Part model, mm, in its own coordinate system. Give positions to 0.01 mm unless a question says otherwise; leave off trailing zeros. Order: outer loops, then holes, each group sorted by start corner. A loop starts at its lowest first (then second) coordinate and runs counter-clockwise, first axis right, second up.
1. Slice it at C-C on y = 235.3. List the corners of the cut face in (x, z), and give its area (3 significant figures).
2. Slice it at B-B on x = -9.25. List the corners of the cut face in (y, z) (3 decimals).
3. Slice it at D-D on x = 18.5. List the corners of the cut face in (y, z) (3 decimals).
4. Drop flat-ended pins along their axis: pin 1 Ø1 at (x, y) = (-17, 235) entering from -Z; pin 2 Ø12 at (x, z) = (-7.5, 15.5) entering from +Y; pin 3 Ø1 at (x, y) = (-5.5, 234.5) entering from +Z. Give the stop position or say it passes through.
5. Slice it at A-A on z = 0. List the corners of the cut face in (x, y) (3 decimals).
6. Probe line 1 (X direction, y = 233.7, z = -1.5); line 2 (X direction, y = 235.85, z = -18); line 3 (Z direction, x = 11, y = 235.1). List the from-to ranges inside material, lowest first.
from build123d import *

# Parameters (mm, degrees)
SKETCH2_R           = 22.5
SKETCH2_R_2         = 2.25
BOSS_EXTRUDE1_DEPTH = 3.175


with BuildPart() as part:
    # Sketch2 → Boss-Extrude1 (new body)
    with BuildSketch(Plane(origin=(0, 236.49, 0), x_dir=(1, 0, 0), z_dir=(0, 1, 0))):
        with Locations(Location((0, 0, 0), (0, 0, 270))):
            Circle(SKETCH2_R)
        with Locations(Location((9.25, 16.02146997, 0), (0, 0, 270))):
            Circle(SKETCH2_R_2, mode=Mode.SUBTRACT)
        with Locations(Location((18.5, 0, 0), (0, 0, 270))):
            Circle(SKETCH2_R_2, mode=Mode.SUBTRACT)
        with Locations(Location((9.25, -16.02146997, 0), (0, 0, 270))):
            Circle(SKETCH2_R_2, mode=Mode.SUBTRACT)
        with Locations(Location((-9.25, -16.02146997, 0), (0, 0, 270))):
            Circle(SKETCH2_R_2, mode=Mode.SUBTRACT)
        with Locations(Location((-18.5, 0, 0), (0, 0, 270))):
            Circle(SKETCH2_R_2, mode=Mode.SUBTRACT)
        with Locations(Location((-9.25, 16.02146997, 0), (0, 0, 270))):
            Circle(SKETCH2_R_2, mode=Mode.SUBTRACT)
    extrude(amount=-BOSS_EXTRUDE1_DEPTH)


solid = part.part
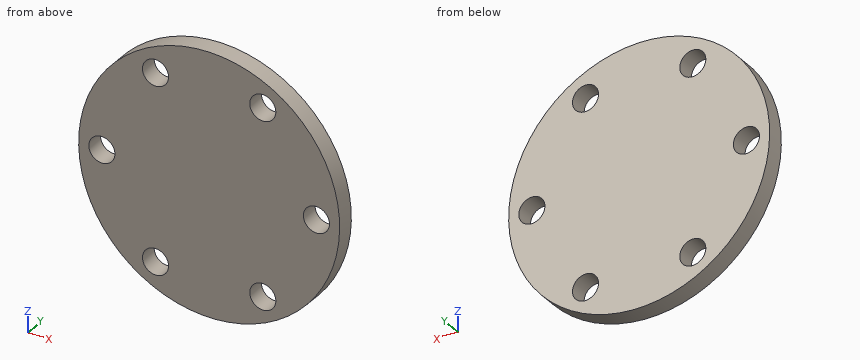
Data:
1. outline: circle Ø45 at (0, 0); hole circle Ø4.5 at (-18.5, 0); hole circle Ø4.5 at (-9.25, -16.02); hole circle Ø4.5 at (-9.25, 16.02); hole circle Ø4.5 at (9.25, -16.02); hole circle Ø4.5 at (9.25, 16.02); hole circle Ø4.5 at (18.5, 0)
1. area: 1,500 mm2
2. outline: (233.315, -20.511) - (236.49, -20.511) - (236.49, -18.271) - (233.315, -18.271) - close; (233.315, -13.771) - (236.49, -13.771) - (236.49, 13.771) - (233.315, 13.771) - close; (233.315, 18.271) - (236.49, 18.271) - (236.49, 20.511) - (233.315, 20.511) - close
3. outline: (233.315, -12.806) - (236.49, -12.806) - (236.49, -2.25) - (233.315, -2.25) - close; (233.315, 2.25) - (236.49, 2.25) - (236.49, 12.806) - (233.315, 12.806) - close
4. pin 1: stops at z = -15.3
4. pin 2: stops at y = 236.49
4. pin 3: stops at z = 21.94
5. outline: (-22.5, 233.315) - (-20.75, 233.315) - (-20.75, 236.49) - (-22.5, 236.49) - close; (-16.25, 233.315) - (16.25, 233.315) - (16.25, 236.49) - (-16.25, 236.49) - close; (20.75, 233.315) - (22.5, 233.315) - (22.5, 236.49) - (20.75, 236.49) - close
6. line 1: x = -22.45 to -20.18, -16.82 to 16.82, 20.18 to 22.45
6. line 2: x = -13.5 to -10.32, -8.18 to 8.18, 10.32 to 13.5
6. line 3: z = -19.63 to -17.44, -14.61 to 14.61, 17.44 to 19.63
